Geometry: final body of the model. Coordinates: model frame, mm. Face numbers are marked on the shaded views. Give positions to 0.01 mm unless a question says otherwise; leave off trailing zeros. Order: outer loops, then holes, each group sorted by start corner. A loop starts at its lowest first (then second) coordinate and runs counter-clockwise, first axis right, second up. Notation, with made-up numbers: (39, -34) -> (82, -34) arc R18 ccw to (82, -1) -> close; hole circle Ø9 at (60.25, -31.5). An arc over 180 degrees is marked (long way). One line per question, with ' | ' between items. Start each with the question number.
(1) Section B-B (y = 0.85). State how many separate pieces and enclosed holes the cut face has, then the cut area to 3 significant figures.
(2) First-contact query: pin 1 Ø1.5 at (x, y) = (-26, 1) entering from +Z; pin 2 Ø0.9 at (y, z) = (1, 21) entering from +X; pin 3 Ø0.9 at (y, z) = (2, -22) entering from -X. Flat tips, straight axial feed; report the tip coordinate or a pass-through.
(3) Section D-D (x = 0). Return loops of the section in (y, z).
(4) Section C-C (z = -20). Return loops of the section in (x, y).
(5) Ray query, L1, parallel to Z at x = 0, y = 2.3; L2, parallel to Z at x = 20, y = 1.3; L3, parallel to Z at x = -33.5, y = 1.5. Return the intervals inside material, ascending.
(6) Section A-A (x = -33.5). Return loops of the section in (y, z), then the cut area to 3 significant figures.
(7) Mould query, pull axis X, two halves, no side actions, for the marked faces 1 and 2. Classes: +X half, -X half, draft (parallel to the pull), parting line (faces both ways), or undercut.
```python
from build123d import *

# Parameters (mm, degrees)
SKETCH_2_W          = 80
SKETCH_2_H          = 15
EXTRUDE_1_DEPTH     = 3
SKETCH_1_R          = 5
EXTRUDE_2_DEPTH     = 2
SKETCH_3_W          = 15
SKETCH_3_H          = 60
EXTRUDE_3_DEPTH     = 3
SKETCH_4_R          = 2.1
CUT_EXTRUDE_4_DEPTH = 4
SKETCH_5_R          = 2.1
CUT_EXTRUDE_5_DEPTH = 4
FILLET_2_R          = 5
SKETCH_6_R          = 1.6
CUT_EXTRUDE_6_DEPTH = 6
FILLET_3_R          = 10


with BuildPart() as part:
    # 草圖2 → 填料-伸長1 (new body)
    with BuildSketch(Plane(origin=(0, 0, 0), x_dir=(1, 0, 0), z_dir=(0, 1, 0))):
        Rectangle(SKETCH_2_W, SKETCH_2_H)
    extrude(amount=EXTRUDE_1_DEPTH)

    # 草圖1 → 填料-伸長2 (add)
    with BuildSketch(Plane(origin=(0, 0, 0), x_dir=(1, 0, 0), z_dir=(0, 1, 0))):
        with Locations((-33.5, 0)):
            Circle(SKETCH_1_R)
        with Locations((33.5, 0)):
            Circle(SKETCH_1_R)
    extrude(amount=-EXTRUDE_2_DEPTH)

    # 草圖3 → 填料-伸長3 (add)
    with BuildSketch(Plane.XZ):
        Rectangle(SKETCH_3_W, SKETCH_3_H)
    extrude(amount=-EXTRUDE_3_DEPTH)

    # 草圖4 → 除料-伸長4 (cut, through all)
    with BuildSketch(Plane.XZ):
        with Locations((0, 20)):
            Circle(SKETCH_4_R)
        with Locations((0, -20)):
            Circle(SKETCH_4_R)
    extrude(amount=-CUT_EXTRUDE_4_DEPTH, mode=Mode.SUBTRACT)

    # 草圖5 → 除料-伸長5 (cut, through all)
    with BuildSketch(Plane.XZ):
        with Locations((-20, 0)):
            Circle(SKETCH_5_R)
        with Locations((20, 0)):
            Circle(SKETCH_5_R)
    extrude(amount=-CUT_EXTRUDE_5_DEPTH, mode=Mode.SUBTRACT)

    # 圓角2
    fillet_2_edges = [part.edges().sort_by_distance(p)[0] for p in [
        (7.5, 1.5, 30),
        (-7.5, 1.5, -30),
        (7.5, 1.5, -30),
        (-7.5, 1.5, 30),
        (40, 1.5, 7.5),
        (-40, 1.5, 7.5),
        (-40, 1.5, -7.5),
        (40, 1.5, -7.5),
    ]]
    fillet(fillet_2_edges, radius=FILLET_2_R)

    # 草圖6 → 除料-伸長6 (cut, through all)
    with BuildSketch(Plane.XZ.offset(2)):
        with Locations((-33.5, 0)):
            Circle(SKETCH_6_R)
        with Locations((33.5, 0)):
            Circle(SKETCH_6_R)
    extrude(amount=-CUT_EXTRUDE_6_DEPTH, mode=Mode.SUBTRACT)

    # 圓角3
    fillet_3_edges = [part.edges().sort_by_distance(p)[0] for p in [
        (7.5, 1.5, -7.5),
        (7.5, 1.5, 7.5),
        (-7.5, 1.5, -7.5),
        (-7.5, 1.5, 7.5),
    ]]
    fillet(fillet_3_edges, radius=FILLET_3_R)


solid = part.part
```
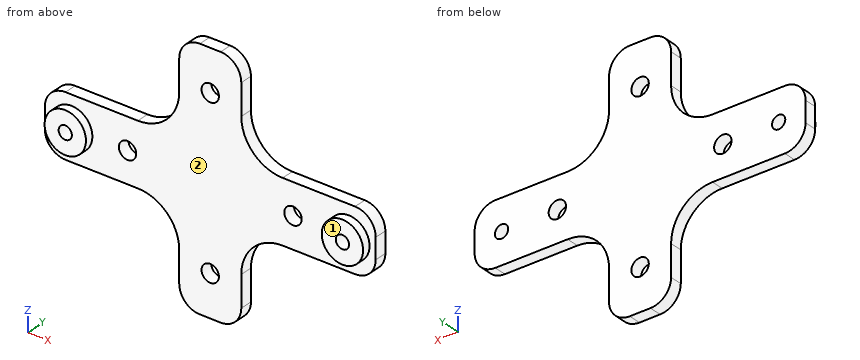
Response:
1) separate pieces: 1 | enclosed holes: 6 | area: 1,850 mm^2
2) pin 1: stops at z = 7.5 | pin 2: stops at x = 7.5 | pin 3: stops at x = -7.5
3) outline: (0, -30) -> (3, -30) -> (3, -22.1) -> (0, -22.1) -> close; (0, -17.9) -> (3, -17.9) -> (3, 17.9) -> (0, 17.9) -> close; (0, 22.1) -> (3, 22.1) -> (3, 30) -> (0, 30) -> close
4) outline: (-7.5, 0) -> (-2.1, 0) -> (-2.1, 3) -> (-7.5, 3) -> close; (2.1, 0) -> (7.5, 0) -> (7.5, 3) -> (2.1, 3) -> close
5) L1: z = -30 to -22.1, -17.9 to 17.9, 22.1 to 30 | L2: z = -7.5 to -2.1, 2.1 to 7.5 | L3: z = -7.5 to -1.6, 1.6 to 7.5
6) outline: (-2, -5) -> (0, -5) -> (0, -7.5) -> (3, -7.5) -> (3, -1.6) -> (-2, -1.6) -> close; (-2, 1.6) -> (3, 1.6) -> (3, 7.5) -> (0, 7.5) -> (0, 5) -> (-2, 5) -> close | area: 49.0 mm^2
7) face 1: draft | face 2: undercut
